from build123d import *

# Parameters (mm, degrees)
F0_R     = 11
F1_DEPTH = 90
F0_R_2   = 12.5
F2_DEPTH = 10
F3_START = 40
F0_R_3   = 13.5
F3_DEPTH = 50
F4_W     = 0.5
F4_H     = 3
F6_R     = 1
F7_SIZE2 = 5
F7_SIZE  = 1


with BuildPart() as f1:
    # F0 (on Top) → F1 (new body)
    with BuildSketch(Plane.XY):
        Circle(F0_R)
    extrude(amount=F1_DEPTH)

    # F0 (on Top) → F2 (join)
    with BuildSketch(Plane.XY):
        Circle(F0_R_2)
        Circle(F0_R, mode=Mode.SUBTRACT)
    extrude(amount=F2_DEPTH)

    # F0 (on Top) → F3 (join)
    with BuildSketch(Plane.XY.offset(F3_START)):
        Circle(F0_R_3)
        Circle(F0_R_2, mode=Mode.SUBTRACT)
        Circle(F0_R_2)
        Circle(F0_R, mode=Mode.SUBTRACT)
    extrude(amount=F3_DEPTH)

    # F4 (on Front) → F5 (revolve)
    with BuildSketch(Plane.XZ):
        with BuildLine():
            Line((-15, 90), (0, 90))
            Line((0, 90), (0, 97.8694483638))
            Line((0, 97.8694483638), (-2.75, 97.8694483638))
            Line((-2.75, 97.8694483638), (-2.75, 99.3694483638))
            Line((-2.75, 99.3694483638), (-3.25, 99.3694483638))
            Line((-3.25, 99.3694483638), (-3.25, 97.8694483638))
            Line((-3.25, 97.8694483638), (-8, 97.8694483638))
            ThreePointArc((-8, 97.8694483638), (-9.5836049581, 98.4817025568), (-10.343494907, 100))
            Line((-10.343494907, 100), (-10.843494907, 100))
            Line((-10.843494907, 100), (-15, 90))
        make_face()
        with Locations((-3, -1.5)):
            Rectangle(F4_W, F4_H)
    revolve(axis=Axis((0, 0, 93.9347241819), (0, 0, 1)))

    # F6
    f6_edges = [f1.edges().sort_by_distance(p)[0] for p in [
        (-12.5, 0, 10),
    ]]
    fillet(f6_edges, radius=F6_R)

    # F7
    f7_edges = [f1.edges().sort_by_distance(p)[0] for p in [
        (-12.5, 0, 0),
    ]]
    f7_side = f1.faces().sort_by_distance((-12.5, 0, 4.5))[0]
    chamfer(f7_edges, length=F7_SIZE, length2=F7_SIZE2, reference=f7_side)


solid = f1.part
Verification items for the finished model (mm, model axes). A direction names the side the tool comes from. Give positions to 0.01 mm unless a question says otherwise; leave off trailing zeros. Loops run counter-clockwise (first coordinate to the right, second up) from the corner with the lowest first, then second, coordinate; pieces in that order, holes last.
1) Set-up check for faces 5 (the flat face through (-5, -10, 40)), 6 (the flat face through (0, 0, 97.869)), 7 (the cylindrical face through (0.596, 2.685, -1.479)): record each of +Z, -Z, +X, -X, +Y, -Y from which the full face is reachable in a straight line by a thin tool's end or side.
2) Sectioned sample at A-A, the plane z = 16. Enter the section's corners in (x, y), then the cut area to 3 significant figures.
3) Thickness scan on line 1 along X through (y, z) = (0, 98.9); line 2 along Y through (x, z) = (0, -1.55); line 3 along Z through (x, y) = (4.5, -2.75). Record the ranges inside material, lowest first.
4) Draft check along Z on faces 1 (the cylindrical face through (11.923, 3.755, 4.944)), 2 (the flat face through (11.18, -7.85, 90)), 3 (the flat face through (3.4, -0.1, 97.869)), 4 (the cylindrical face through (-2.38, -10.74, 24.79)). Enter one of: pulls with the +Z half, pulls with the -Z half, needs draft (parallel to the pull), parting line crosses it, or undercut.
5) Depth check by flat-ended pin: pin 1 Ø2 at (x, z) = (-11, 28.5) entering from +Y; pin 2 Ø11.5 at (x, y) = (-2, -3) entering from +Z; pin 3 Ø1 at (x, z) = (-11, 87.5) entering from -Y. Enter the tip coordinate at first touch or a pass-through.
Answers:
1. face 5: none
1. face 6: +Z
1. face 7: -Z
2. outline: circle Ø22 at (0, 0)
2. area: 380 mm2
3. line 1: x = -11.3 to -9.95, -3.25 to -2.75, 2.75 to 3.25, 9.95 to 11.3
3. line 2: y = -3.25 to -2.75, 2.75 to 3.25
3. line 3: z = 0 to 97.87
4. face 1: needs draft
4. face 2: pulls with the -Z half
4. face 3: pulls with the +Z half
4. face 4: undercut
5. pin 1: stops at y = 4.58
5. pin 2: stops at z = 99.37
5. pin 3: stops at y = -8.49
